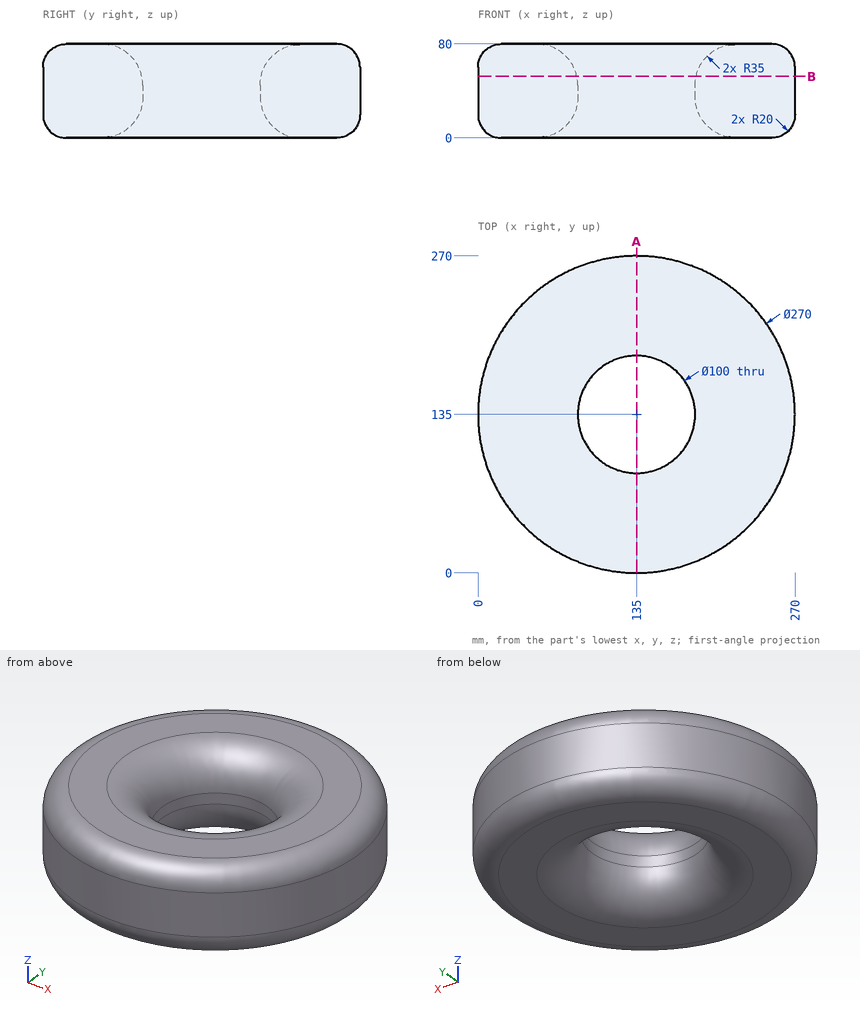
Design review of the part shown in the three views and the two pictorial views. Dimensions are in mm from the part's minimum x, y and z. Give positions to 0.01 mm unless a question says otherwise; leave off trailing zeros. Loops run counter-clockwise (first coordinate to the right, second up) from the corner with the lowest first, then second, coordinate; pieces in that order, holes last. Notation, with made-up numbers: (-8.75, -23.5) -> (23.25, -23.5) arc R4 cw to (23.25, -17.5) -> close; hole circle Ø7 at (46, 35). An arc over 180 degrees is marked (long way). Answer as a JSON object with one key per item and string values. Group by question number.
Q1. Insertion check: pin 1 (3 mm diameter, centred on x = 104.5, z = 62.5, fed in from -Y); pin 2 (2 mm diameter, centred on x = 129.5, z = 11, fed in from -Y); pin 3 (2 mm diameter, centred on y = 37, z = 56, fed in from -X); pin 4 (8 mm diameter, centred on x = 154, y = 97, fed in from +Z). Each pin has a flat end and moves straight along its axis. Give the tip position at first contact, or say it passes through.
Q2. Wall thickness on line 1 along Y through (x, z) = (135, 40); line 2 along Z through (x, y) = (193, 235); line 3 along Y through (x, z) = (112.5, 74.5): over which ranges is each line inside the solid? List them lowest first.
Q3. Take a section at B-B (z = 52.5). Write out the cut boundary in (x, y), plus the area to 3 significant figures.
Q4. Take a section at A-A (x = 135). Write out the cut boundary in (y, z).
Answer below:
{
 "1": {"pin 1": "stops at y = 3.27", "pin 2": "stops at y = 1.78", "pin 3": "stops at x = 41.11", "pin 4": "passes through"},
 "2": {"line 1": "y = 0 to 85, 185 to 270", "line 2": "z = 0.01 to 79.99", "line 3": "y = 8.21 to 72.78, 197.22 to 261.79"},
 "3": {"outline": "circle Ø270 at (135, 135); hole circle Ø101.63 at (135, 135)", "area": "49,100 mm2"},
 "4": {"outline": "(0, 20) arc R20 ccw to (20, 0) -> (50, 0) arc R35 ccw to (85, 35) -> (85, 45) arc R35 ccw to (50, 80) -> (20, 80) arc R20 ccw to (0, 60) -> close; (185, 35) arc R35 ccw to (220, 0) -> (250, 0) arc R20 ccw to (270, 20) -> (270, 60) arc R20 ccw to (250, 80) -> (220, 80) arc R35 ccw to (185, 45) -> close"}
}
